Check sheet for the modelled part. Datum: model origin and axes. Units: mm. Round coordinates to 2 decimals unless told otherwise and drop trailing zeros. Write each loop counter-clockwise with the first axis right and the second up, starting at its lowest first coordinate (ties: lowest second). Pieces come first, ordered by that corner, then holes. Notation, with made-up numbers: (-27.5, 42.25) -> (-2.5, 42.25) arc R21 cw to (-2.5, 76.25) -> close; hole circle Ø9 at (70, -27.5). An arc over 180 degrees is marked (long way). Write item = value, one per line.
from build123d import *

# Parameters (mm, degrees)
F0_W     = 100
F0_H     = 100
F1_DEPTH = 5
F2_SIZE2 = 21.2132
F2_SIZE  = 21.2132
F3_R     = 1.5875
F3_W     = 2.5
F3_H     = 20
F3_W_2   = 20
F3_H_2   = 2.5
F4_DEPTH = 5
F5_R     = 1
F6_W     = 2.5
F6_H     = 15
F7_DEPTH = 5
F8_R     = 1


with BuildPart() as f1:
    # F0 (on Top) → F1 (new body)
    with BuildSketch(Plane.XY):
        Rectangle(F0_W, F0_H)
    extrude(amount=F1_DEPTH)

    # F2
    f2_edges = [f1.edges().sort_by_distance(p)[0] for p in [
        (50, -50, 2.5),
        (50, 50, 2.5),
        (-50, -50, 2.5),
        (-50, 50, 2.5),
    ]]
    chamfer(f2_edges, length=F2_SIZE, length2=F2_SIZE2)

    # F3 (on face) → F4 (cut)
    with BuildSketch(Plane.XY.offset(5)):
        with Locations((-25.251264, 25.251264)):
            Circle(F3_R)
        with Locations((-25.251265, -25.251264)):
            Circle(F3_R)
        with Locations((25.251262, -25.251264)):
            Circle(F3_R)
        with Locations((25.251262, 25.251262)):
            Circle(F3_R)
        with Locations((-18.180197, -18.180194)):
            Circle(F3_R)
        with Locations((18.180192, -18.180194)):
            Circle(F3_R)
        with Locations((18.180192, 18.180192)):
            Circle(F3_R)
        with Locations((-18.180197, 18.180197)):
            Circle(F3_R)
        with Locations((-32.322333, -32.322332)):
            Circle(F3_R)
        with Locations((32.322331, -32.322332)):
            Circle(F3_R)
        with Locations((32.322331, 32.322331)):
            Circle(F3_R)
        with Locations((-32.322333, 32.322332)):
            Circle(F3_R)
        with Locations((-40, 0)):
            Rectangle(F3_W, F3_H)
        with Locations((-45, 0)):
            Circle(F3_R)
        with Locations((0, -40)):
            Rectangle(F3_W_2, F3_H_2)
        with Locations((0, -45)):
            Circle(F3_R)
        with Locations((40, 0)):
            Rectangle(F3_W, F3_H)
        with Locations((45, 0)):
            Circle(F3_R)
        with Locations((0, 45)):
            Circle(F3_R)
        with Locations((0, 40)):
            Rectangle(F3_W_2, F3_H_2)
    extrude(amount=-F4_DEPTH, mode=Mode.SUBTRACT)

    # F5
    f5_edges = [f1.edges().sort_by_distance(p)[0] for p in [
        (-41.25, 10, 2.5),
        (-10, -38.75, 2.5),
        (38.75, 10, 2.5),
        (-10, 41.25, 2.5),
        (10, -38.75, 2.5),
        (41.25, 10, 2.5),
        (-38.75, 10, 2.5),
        (10, 41.25, 2.5),
        (41.25, -10, 2.5),
        (10, -41.25, 2.5),
        (10, 38.75, 2.5),
        (-38.75, -10, 2.5),
        (-10, 38.75, 2.5),
        (38.75, -10, 2.5),
        (-41.25, -10, 2.5),
        (-10, -41.25, 2.5),
    ]]
    fillet(f5_edges, radius=F5_R)

    # F6 (on face) → F7 (cut)
    with BuildSketch(Plane.XY.offset(5)):
        Polygon((7.499998, 16.930197), (7.499998, 19.430197), (-2e-06, 19.430197), (-7.500002, 19.430197), (-7.500002, 18.180197), (-7.500002, 16.930197), align=None)
        with Locations((-18.180197, -1e-06)):
            Rectangle(F6_W, F6_H)
        Polygon((7.499998, -19.430199), (7.499998, -16.930199), (-7.500002, -16.930199), (-7.500002, -19.430199), (-2e-06, -19.430199), align=None)
        with Locations((18.180192, -1e-06)):
            Rectangle(F6_W, F6_H)
        Polygon((-27.824168, -1e-06), (-27.824168, 8.499999), (-30.324168, 8.499999), (-30.324168, -8.500001), (-27.824168, -8.500001), align=None)
        Polygon((8.499998, -29.430194), (8.499998, -26.930194), (-2e-06, -26.930194), (-8.500002, -26.930194), (-8.500002, -29.430194), align=None)
        Polygon((29.430192, -8.499999), (29.430192, 8.500001), (26.930192, 8.500001), (26.930192, 1e-06), (26.930192, -8.499999), align=None)
        Polygon((8.499998, 26.930197), (8.499998, 29.430197), (-8.500002, 29.430197), (-8.500002, 26.930197), (-2e-06, 26.930197), align=None)
    extrude(amount=-F7_DEPTH, mode=Mode.SUBTRACT)

    # F8
    f8_edges = [f1.edges().sort_by_distance(p)[0] for p in [
        (-30.324168, 8.499999, 2.5),
        (-19.430197, 7.499999, 2.5),
        (-8.500002, 29.430197, 2.5),
        (-7.500002, 19.430197, 2.5),
        (-7.500002, -16.930199, 2.5),
        (-8.500002, -26.930194, 2.5),
        (16.930192, 7.499999, 2.5),
        (26.930192, 8.500001, 2.5),
        (8.499998, 29.430197, 2.5),
        (7.499998, 19.430197, 2.5),
        (-27.824168, 8.499999, 2.5),
        (-16.930197, 7.499999, 2.5),
        (29.430192, 8.500001, 2.5),
        (19.430192, 7.499999, 2.5),
        (7.499998, -16.930199, 2.5),
        (8.499998, -26.930194, 2.5),
        (29.430192, -8.499999, 2.5),
        (19.430192, -7.500001, 2.5),
        (7.499998, -19.430199, 2.5),
        (8.499998, -29.430194, 2.5),
        (7.499998, 16.930197, 2.5),
        (8.499998, 26.930197, 2.5),
        (-27.824168, -8.500001, 2.5),
        (-16.930197, -7.500001, 2.5),
        (-7.500002, -19.430199, 2.5),
        (-8.500002, -29.430194, 2.5),
        (-30.324168, -8.500001, 2.5),
        (-19.430197, -7.500001, 2.5),
        (16.930192, -7.500001, 2.5),
        (26.930192, -8.499999, 2.5),
        (-8.500002, 26.930197, 2.5),
        (-7.500002, 16.930197, 2.5),
    ]]
    fillet(f8_edges, radius=F8_R)


solid = f1.part
(1) Sectioned sample at A-A on x = 45. Enter the section's corners in (y, z).
Worked answers:
outline = (-33.79, 0) -> (-1.59, 0) -> (-1.59, 5) -> (-33.79, 5) -> close; (1.59, 0) -> (33.79, 0) -> (33.79, 5) -> (1.59, 5) -> close
(2) Release check for a two-part mould opening along Y. For faces 1 (the flat face through (-50, 0, 2)), 2 (the flat face through (19.43, 0, 3)), 3 (the flat face through (0, 50, 2)) record: pulls with the +Y half, pulls with the -Y half, needs draft (parallel to the pull), parting line crosses it, or undercut.
Worked answers:
face_1 = needs draft
face_2 = undercut
face_3 = pulls with the +Y half
(3) Sectioned sample at B-B on y = 0. Count the separate pieces of the cut face and the enclosed holes in it, then the cut area to 3 significant figures.
Worked answers:
separate_pieces = 9
enclosed_holes = 0
area = 393 mm²
(4) Go/stop test with flat-tipped pins: P1, Ø1, axis at x = 35.5, z = 2, coming from the +Y side; P2, Ø3, axis at x = -25.25, y = -25.25, coming from the -Z side; P3, Ø1, axis at y = -32.5, z = 2.5, coming from the +X side. Record where each tip stops, or that it passes through.
Worked answers:
P1 = 43.79
P2 = through
P3 = 46.79
(5) Material ranges on L1, parallel to X at y = 9, z = 1; L2, parallel to Y at x = -25, z = 2.15; L3, parallel to X at y = 8, z = 1.1, recorded low to high. Write a range as [from, to].
Worked answers:
L1 = [-50, -41.25], [-38.75, 38.75], [41.25, 50]
L2 = [-50, -26.82], [-23.68, 23.68], [26.82, 50]
L3 = [-50, -41.25], [-38.75, -30.19], [-27.96, 27.06], [29.3, 38.75], [41.25, 50]
